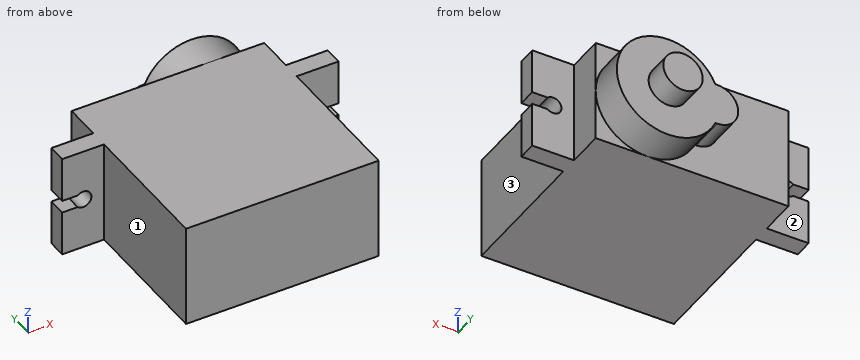
```python
from build123d import *

# Parameters (mm, degrees)
SKETCH_1_W          = 23
SKETCH_1_H          = 12.3
EXTRUDE_1_DEPTH     = 23.3
SKETCH_3_W          = 5
SKETCH_3_H          = 2.2
EXTRUDE_2_DEPTH     = 12.3
CUT_EXTRUDE_1_DEPTH = 36.951356024
EXTRUDE_3_DEPTH     = 4.3
SKETCH_6_R          = 2.35
EXTRUDE_4_DEPTH     = 3


with BuildPart() as part:
    # Эскиз1 → Бобышка-Вытянуть1 (new body)
    with BuildSketch(Plane(origin=(0, 0, 0), x_dir=(1, 0, 0), z_dir=(0, 1, 0))):
        with Locations((11.5, 6.15)):
            Rectangle(SKETCH_1_W, SKETCH_1_H)
    extrude(amount=EXTRUDE_1_DEPTH)

    # Эскиз3 → Бобышка-Вытянуть2 (add)
    with BuildSketch(Plane.XY):
        with Locations((25.5, 17.8)):
            Rectangle(SKETCH_3_W, SKETCH_3_H)
    extrude_2 = extrude(amount=-EXTRUDE_2_DEPTH)

    # Эскиз4 → Вырез-Вытянуть1 (cut, through all)
    with BuildSketch(Plane(origin=(0, 18.9, 0), x_dir=(1, 0, 0), z_dir=(0, 1, 0))):
        with BuildLine():
            Line((28, 6.15), (28, 6.9))
            Line((28, 6.9), (26.161437828, 6.9))
            ThreePointArc((26.161437828, 6.9), (24.5, 6.15), (26.161437828, 5.4))
            Line((26.161437828, 5.4), (28, 5.4))
            Line((28, 5.4), (28, 6.15))
        make_face()
    cut_extrude_1 = extrude(amount=-CUT_EXTRUDE_1_DEPTH, mode=Mode.SUBTRACT)

    # Зеркальное отражение2: Бобышка-Вытянуть2, Вырез-Вытянуть1 across plane
    add(extrude_2.mirror(Plane.ZY.offset(-11.5)))
    add(cut_extrude_1.mirror(Plane.ZY.offset(-11.5)), mode=Mode.SUBTRACT)

    # Эскиз5 → Бобышка-Вытянуть3 (add)
    with BuildSketch(Plane(origin=(0, 23.3, 0), x_dir=(1, 0, 0), z_dir=(0, 1, 0))):
        with BuildLine():
            Line((11, 3.65), (11.231058819, 3.65))
            ThreePointArc((11.231058819, 3.65), (23, 6.15), (11.231058819, 8.65))
            Line((11.231058819, 8.65), (11, 8.65))
            ThreePointArc((11, 8.65), (8.5, 6.15), (11, 3.65))
        make_face()
    extrude(amount=EXTRUDE_3_DEPTH)

    # Эскиз6 → Бобышка-Вытянуть4 (add)
    with BuildSketch(Plane(origin=(0, 27.6, 0), x_dir=(1, 0, 0), z_dir=(0, 1, 0))):
        with Locations(Location((16.85, 6.15, 0), (0, 0, 270))):
            Circle(SKETCH_6_R)
    extrude(amount=EXTRUDE_4_DEPTH)


solid = part.part
```
Can you work these out from the model? Positions are in its coordinate system, mm. Face numbers are marked on the shaded views. A direction names the side the tool comes from. Round coordinates to 2 decimals unless told otherwise and drop trailing zeros. Loops run counter-clockwise (first coordinate to the right, second up) from the corner with the lowest first, then second, coordinate; pieces in that order, holes last. Notation, with made-up numbers: M 8.5,83.5 L 43.5,83.5 A26 ccw 43.5,109.5 Z; hole C 81,69 d10. An arc over 180 degrees is marked long. Answer in a Markdown table with one row per item.
1. If we section it at D-D, the plane x = 9.5: Please give me the cut outline in (y, z).
Established:
| item | result |
|---|---|
| outline | M 0,-12.3 L 23.3,-12.3 L 23.3,-8.15 L 27.6,-8.15 L 27.6,-4.15 L 23.3,-4.15 L 23.3,0 L 0,0 Z |
2. If we section it at C-C, the plane y = 24.5: Please give me the cut outline in (x, z).
Established:
| item | result |
|---|---|
| outline | M 11,-8.65 L 11.23,-8.65 A6.15 ccw long 11.23,-3.65 L 11,-3.65 A2.5 ccw Z |
3. On a 3-axis mill with a long thin cutter (end or side, diameter ignored), from which of +Z, -Z, +X, -X, +Y, -Y can I reach the whole of each face in a straight line? I mean the marked faces 1, 2 and 3. Say none if no direction works.
Established:
| item | result |
|---|---|
| face 1 | +Z, -Z, -X, -Y |
| face 2 | +Z, -Z, -X, +Y |
| face 3 | +Z, -Z, +X, -Y |
4. If we section it at A-A, the plane x = -2.5: Please give me the cut outline in (y, z).
Established:
| item | result |
|---|---|
| outline | M 16.7,-12.3 L 18.9,-12.3 L 18.9,-7.15 L 16.7,-7.15 Z; M 16.7,-5.15 L 18.9,-5.15 L 18.9,0 L 16.7,0 Z |
5. If we section it at B-B, the plane z = -9.5: Please give me the cut outline in (x, y).
Established:
| item | result |
|---|---|
| outline | M -5,16.7 L 0,16.7 L 0,0 L 23,0 L 23,16.7 L 28,16.7 L 28,18.9 L 23,18.9 L 23,23.3 L 22.01,23.3 L 22.01,27.6 L 11.69,27.6 L 11.69,23.3 L 0,23.3 L 0,18.9 L -5,18.9 Z |
6. I'm going to push flat-ended pins straight in: pin 1 Ø6 at (y, z) = (25, -7) entering from +X; pin 2 Ø1.8 at (x, z) = (20.5, -2.5) entering from +Y; pin 3 Ø2 at (y, z) = (22, -3.5) entering from -X; pin 4 Ø0.9 at (x, y) = (-4, 18) entering from +Z. Where does each tip first touch, or does it pass through?
Established:
| item | result |
|---|---|
| pin 1 | x = 23 |
| pin 2 | y = 27.6 |
| pin 3 | x = 0 |
| pin 4 | z = 0 |
7. Please list where these lines run through material, in increasing order: line 1 (Z direction, x = -2.5, y = 18.1); line 2 (Y direction, x = 5, z = -9.75); line 3 (Y direction, x = 14.5, z = -10.25). Write a range as from..to.
Established:
| item | result |
|---|---|
| line 1 | -12.3..-7.15, -5.15..0 |
| line 2 | 0..23.3 |
| line 3 | 0..27.6 |
